from build123d import *

# Parameters (mm, degrees)
F0_R     = 38.1
F1_DEPTH = 76.2
F3_DEPTH = 71.882
F4_DEPTH = 64.77


with BuildPart() as f1:
    # F0 (on Top) → F1 (new body)
    with BuildSketch(Plane.XY):
        Circle(F0_R)
    extrude(amount=F1_DEPTH)

    # F2 (on Front) → F3 (cut)
    with BuildSketch(Plane.XZ):
        Polygon((-49.077209, 0), (-38.439587, 0), (0, 76.531306), (37.743848, 0), (45.744851, 0), (45.744851, 81.064962), (-51.657092, 81.064962), align=None)
    extrude(amount=F3_DEPTH, mode=Mode.SUBTRACT)

    # F2 (on Front) → F4 (cut)
    with BuildSketch(Plane.XZ):
        Polygon((-49.077209, 0), (-38.439587, 0), (0, 76.531306), (37.743848, 0), (45.744851, 0), (45.744851, 81.064962), (-51.657092, 81.064962), align=None)
    extrude(amount=-F4_DEPTH, mode=Mode.SUBTRACT)


solid = f1.part
Check sheet for the modelled part. Datum: model origin and axes. Units: mm. Give positions to 0.01 mm unless a question says otherwise; leave off trailing zeros. Write each loop counter-clockwise with the first axis right and the second up, starting at its lowest first coordinate (ties: lowest second). Pieces come first, ordered by that corner, then holes. Notation, with made-up numbers: (-25.75, 48.5) -> (-17.75, 48.5) arc R22 ccw to (-17.75, 72.5) -> close; hole circle Ø1 at (3.5, 16). An arc over 180 degrees is marked (long way). Use one line per item in the form item = value. Start each with the question number.
1. Section check D-D (y = 10). Record the cut outline in (x, z).
2. Go/stop test with flat-tipped pins: P1, Ø4, axis at y = -10, z = 61.5, coming from the +X side; P2, Ø12, axis at x = 8, z = 56, coming from the +Y side; P3, Ø12, axis at y = -5.5, z = 39, coming from the -X side. Record where each tip stops, or that it passes through.
3. Thickness scan on line 1 along Y through (x, z) = (-1, 15.5); line 2 along X through (y, z) = (-20, 49); line 3 along X through (y, z) = (4, 25). Record the ranges inside material, lowest first. Write a range as from..to.
4. Section check A-A (y = 0). Record the cut outline in (x, z).
5. Section check C-C (z = 63.5). Record the cut outline in (x, y).
6. Section check B-B (x = 21.5). Record the cut outline in (y, z).
Conclusion:
q1.outline = (-36.76, 0) -> (36.76, 0) -> (36.76, 1.99) -> (0.16, 76.2) -> (-0.17, 76.2) -> (-36.76, 3.34) -> close
q2.P1 = 8.4
q2.P2 = 38.05
q2.P3 = -21.86
q3.line_1 = -38.09..38.09
q3.line_2 = -13.83..13.58
q3.line_3 = -25.88..25.41
q4.outline = (-38.1, 0) -> (37.74, 0) -> (0.16, 76.2) -> (-0.17, 76.2) -> (-38.1, 0.68) -> close
q5.outline = (-6.55, -37.53) arc R38.1 ccw to (6.43, -37.55) -> (6.43, 37.55) arc R38.1 ccw to (-6.55, 37.53) -> close
q6.outline = (-31.45, 0) -> (31.45, 0) -> (31.45, 32.94) -> (-31.45, 32.94) -> close
